Geometry: final body of the model. Coordinates: model frame, mm. Round coordinates to 2 decimals unless told otherwise and drop trailing zeros. Write each loop counter-clockwise with the first axis right and the second up, starting at its lowest first coordinate (ties: lowest second). Pieces come first, ordered by that corner, then holes. Notation, with made-up numbers: M -27.75,36 L 22.25,36 A20 cw 22.25,58 Z; hole C 35,24.25 d11. An arc over 180 degrees is marked long. Use one line per item in the form item = value. Start each with the question number.
from build123d import *

# Parameters (mm, degrees)
F0_R     = 15
F1_DEPTH = 3
F2_R     = 1.5
F3_DEPTH = 3
F4_R     = 2.5
F5_DEPTH = 3


with BuildPart() as f1:
    # F0 (on Front) → F1 (new body)
    with BuildSketch(Plane.XZ):
        Circle(F0_R)
    extrude(amount=F1_DEPTH)

    # F2 (on face) → F3 (cut, through all)
    with BuildSketch(Plane.XZ.offset(3)):
        with Locations((0, 12)):
            Circle(F2_R)
    extrude(amount=-F3_DEPTH, mode=Mode.SUBTRACT)

    # F4 (on face) → F5 (cut, through all)
    with BuildSketch(Plane.XZ.offset(3)):
        Circle(F4_R)
    extrude(amount=-F5_DEPTH, mode=Mode.SUBTRACT)


solid = f1.part
1. Pull-direction query (Z, two-part tool) for faces 1 (the face through (3, 0, 0)), 2 (the face through (-0.325, -1.521, 10.536)), 3 (the face through (-0.54, -1.52, -2.44)), 4 (the face through (-14.985, -1.479, 0.66)); classes: released by +Z, released by -Z, zero draft, split by the parting line, or undercut.
2. Section query C-C (y = -2.4). Return loops of the section in (x, z).
3. Section query B-B (x = 0). Return loops of the section in (y, z).
4. Section query A-A (z = 0). Return loops of the section in (x, y), then the cut area to 3 significant figures.
5. Section query D-D (z = 12). Return loops of the section in (x, y).
6. Ray query, probe 1 along Z at (x, y) = (0, -2); probe 2 along X at (y, z) = (-2.3, 2); probe 3 along Z at (x, y) = (-9, -2.3). Return the intervals inside material, ascending.
7. Contact query for flat-ended pins moving along their axis: pin 1 (4 mm diameter, centred on x = 0, z = 12, fed in from +Y); pin 2 (1 mm diameter, centred on y = -2.5, z = 3.5, fed in from -X); pin 3 (1 mm diameter, centred on y = -0.5, z = 7.5, fed in from +X); pin 4 (1.5 mm diameter, centred on x = -4, y = -1.5, fed in from +Z). Output: stop coordinate, or through.
Checks:
q1.face_1 = zero draft
q1.face_2 = undercut
q1.face_3 = undercut
q1.face_4 = split by the parting line
q2.outline = C 0,0 d30; hole C 0,0 d5; hole C 0,12 d3
q3.outline = M -3,-15 L 0,-15 L 0,-2.5 L -3,-2.5 Z; M -3,2.5 L 0,2.5 L 0,10.5 L -3,10.5 Z; M -3,13.5 L 0,13.5 L 0,15 L -3,15 Z
q4.outline = M -15,-3 L -2.5,-3 L -2.5,0 L -15,0 Z; M 2.5,-3 L 15,-3 L 15,0 L 2.5,0 Z
q4.area = 75.0 mm^2
q5.outline = M -9,-3 L -1.5,-3 L -1.5,0 L -9,0 Z; M 1.5,-3 L 9,-3 L 9,0 L 1.5,0 Z
q6.probe_1 = -15 to -2.5, 2.5 to 10.5, 13.5 to 15
q6.probe_2 = -14.87 to -1.5, 1.5 to 14.87
q6.probe_3 = -12 to 12
q7.pin_1 = 0
q7.pin_2 = -14.7
q7.pin_3 = 13.27
q7.pin_4 = 14.64
